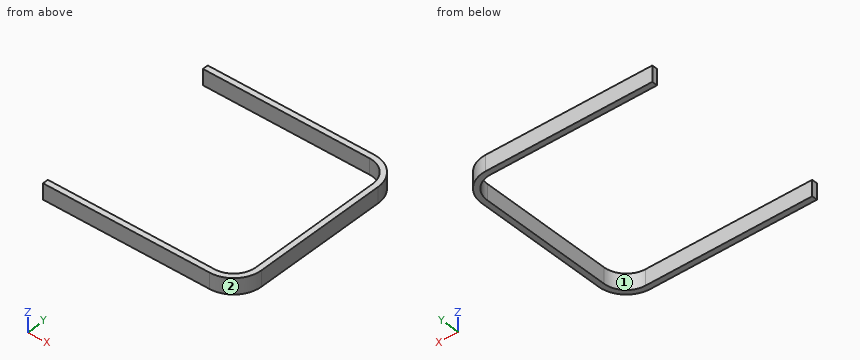
```python
from build123d import *

# Parameters (mm, degrees)
F1_W = 1.589909
F1_H = 4.523729


with BuildPart() as f2:
    # F2: sweep along a path in F0
    with BuildLine(Plane.XY) as f2_path:
        Line((0, 0), (47.690287, 0))
        ThreePointArc((47.690287, 0), (52.180415, 1.859872), (54.040287, 6.35))
        Line((54.040287, 6.35), (54.040287, 44.896792))
        ThreePointArc((54.040287, 44.896792), (52.180415, 49.38692), (47.690287, 51.246792))
        Line((47.690287, 51.246792), (0, 51.246792))
    # F1 (on Right) → F2 (sweep)
    with BuildSketch(Plane.YZ):
        with Locations((-0.794955, 2.261864)):
            Rectangle(F1_W, F1_H)
    sweep(path=f2_path.line)


solid = f2.part
```
Verification items for the finished model (mm, model axes). Face numbers are marked on the shaded views. Round coordinates to 2 decimals unless told otherwise and drop trailing zeros. Write each loop counter-clockwise with the first axis right and the second up, starting at its lowest first coordinate (ties: lowest second). Pieces come first, ordered by that corner, then holes.
1. Draft check along Y on the marked faces 1 and 2. Enter one of: +Y half, -Y half, draft (parallel to the pull), parting line (faces both ways), or undercut.
2. Gauge pin test, flat end, axial feed: P1, Ø2, axis at y = 5, z = 2, coming from the -X side. Record the tip position at first contact, or that the pin passes through.
3. Section check B-B on z = 2.35. Enter the section's corners in (x, y).
4. Section check D-D on y = 5. Enter the section's corners in (x, z), plus the area to 3 significant figures.
5. Section check A-A on x = 18. Enter the section's corners in (y, z), plus the area to 3 significant figures.
6. Section check C-C on y = 42.5. Enter the section's corners in (x, z), plus the area to 3 significant figures.
7. Scan lines: L1, parallel to Y at x = 33, z = 3.9; L2, parallel to X at y = 38.5, z = 1.05. Record each from-to range of solid material in increasing order.
Answer:
1. face 1: undercut
1. face 2: -Y half
2. P1: stops at x = 53.59
3. outline: (0, -1.59) - (47.69, -1.59) arc R7.94 ccw to (55.63, 6.35) - (55.63, 44.9) arc R7.94 ccw to (47.69, 52.84) - (0, 52.84) - (0, 51.25) - (47.69, 51.25) arc R6.35 cw to (54.04, 44.9) - (54.04, 6.35) arc R6.35 cw to (47.69, 0) - (0, 0) - close
4. outline: (53.9, 0) - (55.51, 0) - (55.51, 4.52) - (53.9, 4.52) - close
4. area: 7.33 mm2
5. outline: (-1.59, 0) - (0, 0) - (0, 4.52) - (-1.59, 4.52) - close; (51.25, 0) - (52.84, 0) - (52.84, 4.52) - (51.25, 4.52) - close
5. area: 14.4 mm2
6. outline: (54.04, 0) - (55.63, 0) - (55.63, 4.52) - (54.04, 4.52) - close
6. area: 7.19 mm2
7. L1: y = -1.59 to 0, 51.25 to 52.84
7. L2: x = 54.04 to 55.63
